Part model, mm, in its own coordinate system. Face numbers are marked on the shaded views. Coordinates: 2 decimals unless noted, no trailing zeros. Write each loop counter-clockwise with the first axis right and the second up, starting at its lowest first coordinate (ties: lowest second). Pieces come first, ordered by that corner, then holes. Notation, with made-up numbers: (34.5, -22.5) -> (49.5, -22.5) arc R32 cw to (49.5, 7.5) -> close; hole circle Ø11 at (32, -19.75). An arc over 180 degrees is marked (long way). One line per question, with ' | ' between items. Start each with the question number.
Item 1: Probe probe 1 along Z at (x, y) = (0, 1.65); probe 2 along Z at (x, y) = (0, 21); probe 3 along Y at (x, z) = (-1, -25). List the from-to ranges inside material, lowest first. Write a range as [from, to].
Item 2: Saw through at A-A (z = 0). List the corners of the cut face in (x, y), and give its area (3 significant figures).
Item 3: Two-plate mould, pull along X, no slides. Class the marked faces 1, 2, 3 and 4: pulls with the +X half, pulls with the -X half, needs draft (parallel to the pull), parting line crosses it, or undercut.
Item 4: Saw through at D-D (z = 50). List the corners of the cut face in (x, y).
Item 5: Saw through at B-B (y = 4.5). List the corners of the cut face in (x, z), and give its area (3 significant figures).
Item 6: Pin check, flat tips, straight feed: pin 1 (4 mm diameter, centred on x = -0.5, z = -40.5, fed in from +Y); pin 2 (4 mm diameter, centred on y = 12.5, z = 18, fed in from -X); pin 3 (2.5 mm diameter, centred on x = 35.36, z = -35.36, fed in from +Y); pin 4 (5 mm diameter, centred on x = -41, y = 24.5, fed in from -Z). Stop position of each tip, or through.
Item 7: Saw through at C-C (x = -50). List the corners of the cut face in (y, z), and give its area (3 significant figures).
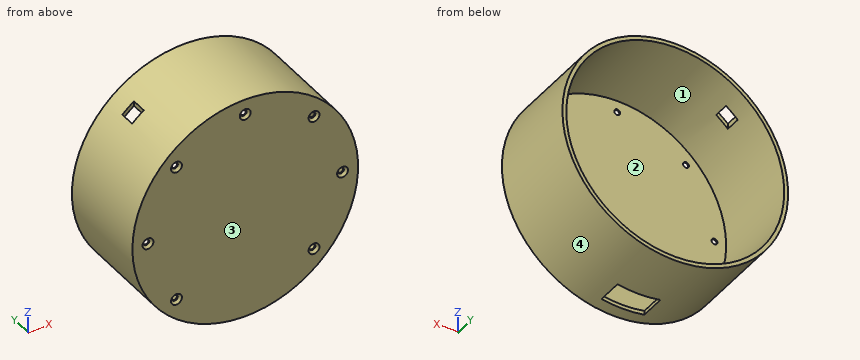
Autodesk Inventor part; units mm, degrees
ref_plane "РабПлоскость2" through (0, 49.211, 0) normal (0, 1, 0) x (1, 0, 0)
ref_plane "РабПлоскость6" through (-79.4555, 0, 0) normal (0, 0, -1) x (1, 0, 0)
ref_plane "YZ Plane" through (0, 0, 0) normal (1, 0, 0) x (0, 1, 0)
sketch "Эскиз1" plane through (0, 0, 0) normal (0, 1, 0) x (-1, 0, 0)
  circle A0 centre (0, 0) radius 58
  line L0 (79.4555, 0) -> (-79.4555, 0)
  line L1 (0, -106.6382) -> (0, 90.6575)
  dimension "d0" = 116
extrude "Выдавливание1" add sketch "Эскиз1" along normal blind 2
sketch "Эскиз2" plane through (0, 0, 0) normal (0, -1, 0) x (1, 0, 0)
  circle A0 centre (0, 0) radius 57
  line L0 (0, -103.8803) -> (0, 88.3129)
  line L1 (-79.4555, 0) -> (79.4555, 0)
  circle A1 centre (0, 0) radius 50
  circle A2 centre (0, -50) radius 1.5
  circle A3 centre (50, 0) radius 1.5
  circle A4 centre (0, 50) radius 1.5
  circle A5 centre (-50, 0) radius 1.5
  circle A6 centre (35.3553, -35.3553) radius 1.5
  circle A7 centre (50, 0) radius 1.5
  circle A8 centre (35.3553, 35.3553) radius 1.5
  circle A9 centre (0, 50) radius 1.5
  circle A10 centre (-35.3553, 35.3553) radius 1.5
  circle A11 centre (-50, 0) radius 1.5
  circle A12 centre (-35.3553, -35.3553) radius 1.5
  dimension "d22" = 3
  dimension "d23" = 3
  dimension "d26" = 3
  dimension "d30" = 360
  dimension "d84" = 114
sketch "Эскиз6" plane through (0, 2, 0) normal (0, 1, 0) x (1, 0, 0)
  circle A0 centre (0, 0) radius 58
  dimension "d85" = 116
ref_plane "РабПлоскость2" through (0, 49.211, 0) normal (0, 1, 0) x (1, 0, 0)
sketch "Эскиз7" plane through (0, 49.211, 0) normal (0, 1, 0) x (1, 0, 0)
  circle A0 centre (0, 0) radius 58
  dimension "d86" = 116
loft "Лофт1" add profiles "Эскиз7", "Эскиз6"
sketch "Эскиз8" plane through (0, 49.211, 0) normal (0, 1, 0) x (1, 0, 0)
  circle A0 centre (0, 0) radius 56
  dimension "d83" = 112
extrude "Выдавливание9" cut sketch "Эскиз8" against normal blind 47.211
ref_plane "РабПлоскость6" through (-79.4555, 0, 0) normal (0, 0, -1) x (1, 0, 0)
sketch "Эскиз10" plane through (-79.4555, 0, 0) normal (0, 0, -1) x (1, 0, 0)
  line L0 (137.4555, -49.211) -> (21.4555, -49.211)
  line L1 (79.4555, 0) -> (79.4555, -49.211)
  line L2 (68.4555, -6.6479) -> (90.4555, -6.6479)
  line L3 (90.4555, -6.6479) -> (90.4555, -19.6479)
  line L4 (90.4555, -19.6479) -> (68.4555, -19.6479)
  line L5 (68.4555, -19.6479) -> (68.4555, -6.6479)
  line L6 (60.4965, -15.4479) -> (98.4145, -15.4479)
  line L7 (98.4145, -15.4479) -> (98.4145, -23.8479)
  line L8 (98.4145, -23.8479) -> (60.4965, -23.8479)
  line L9 (60.4965, -23.8479) -> (60.4965, -15.4479)
  circle A0 centre (60.4965, -15.4479) radius 1.15
  circle A1 centre (98.4145, -15.4479) radius 1.15
  line L10 (45.8699, -29.3481) -> (39.8699, -29.3481)
  line L11 (39.8699, -29.3481) -> (39.8699, -37.3481)
  line L12 (39.8699, -37.3481) -> (45.8699, -37.3481)
  line L13 (45.8699, -37.3481) -> (45.8699, -29.3481)
  point P0 (79.4555, 0)
  dimension "d94" = 22
  dimension "d95" = 13
  dimension "d101" = 37.918
  dimension "d102" = 8.4
  dimension "d103" = 2.3
  dimension "d104" = 2.3
  dimension "d114" = 6
  dimension "d115" = 8
extrude "Выдавливание11" cut sketch "Эскиз10" along normal blind 60 contours L2 L3 L6 L1 | L1 L6 L5 L2 | L6 L3 L4 L1 | L1 L4 L5 L6
hole "Отверстие1" at (0, 0, 50) at (-35.3553, 0, 35.3553) at (35.3553, 0, 35.3553) at (50, 0, 0) at (35.3553, 0, -35.3553) at (-35.3553, 0, -35.3553) at (-50, 0, 0) direction (0, 1, 0) diameter 3 end through all countersink diameter 5.6 countersink angle 90
extrude "Выдавливание13" cut sketch "Эскиз10" against normal blind 60 contours L13 L12 L11 L10
properties part number "caseTop" material "Пластик АБС"
From the geometry:
1) probe 1: [-58, 48.5], [51.5, 58] | probe 2: [-58, -56], [56, 58] | probe 3: [0, 2]
2) outline: (-58, 0) -> (-52.8, 0) -> (-51.5, 1.3) -> (-51.5, 2) -> (-56, 2) -> (-56, 49.21) -> (-58, 49.21) -> close; (-48.5, 1.3) -> (-47.2, 0) -> (47.2, 0) -> (48.5, 1.3) -> (48.5, 2) -> (-48.5, 2) -> close; (51.5, 1.3) -> (52.8, 0) -> (58, 0) -> (58, 49.21) -> (56, 49.21) -> (56, 2) -> (51.5, 2) -> close | area: 405 mm2
3) face 1: undercut | face 2: undercut | face 3: needs draft | face 4: parting line crosses it
4) outline: (-29.39, 0) -> (-2.8, 0) -> (-1.5, 1.3) -> (-1.5, 2) -> (-25.22, 2) -> (-25.22, 49.21) -> (-29.39, 49.21) -> close; (1.5, 1.3) -> (2.8, 0) -> (29.39, 0) -> (29.39, 49.21) -> (25.22, 49.21) -> (25.22, 2) -> (1.5, 2) -> close
5) outline: circle Ø116 at (0, 0); hole circle Ø112 at (0, 0) | area: 716 mm2
6) pin 1: y = 2 | pin 2: x = -55.75 | pin 3: through | pin 4: z = -43.38
7) outline: (0, -29.39) -> (49.21, -29.39) -> (49.21, -25.22) -> (2, -25.22) -> (2, -1.5) -> (1.3, -1.5) -> (0, -2.8) -> close; (0, 2.8) -> (1.3, 1.5) -> (2, 1.5) -> (2, 25.22) -> (49.21, 25.22) -> (49.21, 29.39) -> (0, 29.39) -> close | area: 504 mm2
